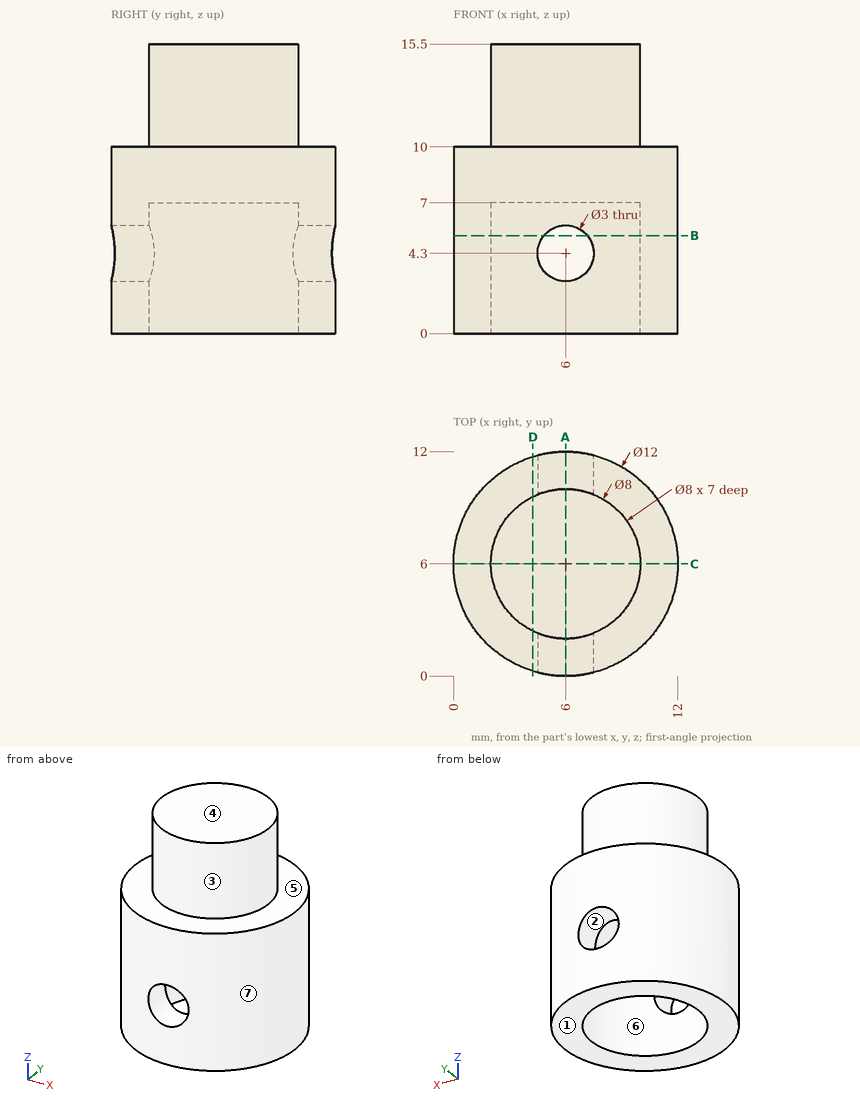
Geometry check sheet. Reference: drawing and pictorial views, mm from the part's lowest x, y, z. A direction names the side the tool comes from. Give positions to 0.01 mm unless a question says otherwise; leave off trailing zeros. Loops run counter-clockwise (first coordinate to the right, second up) from the corner with the lowest first, then second, coordinate; pieces in that order, holes last. Notation, with made-up numbers: M -28,41.5 L -12,41.5 A14 ccw -12,49.5 Z; hole C 41.5,70.5 d8. An arc over 180 degrees is marked long. Use a Markdown table: item, result. Add a question column.
Q1. Sectioned sample at A-A, the plane x = 6. Record the cut outline in (y, z), then the cut area to 3 significant figures.
Q2. Sectioned sample at D-D, the plane x = 4.25. Record the cut outline in (y, z).
Q3. Tool access check on the marked faces 5, 6 and 7. Record the directions out of +Z, -Z, +X, -X, +Y, -Y that give a thin tool (end or side, any length) a straight path to the whole face; none if there is none.
Q4. Go/stop test with flat-tipped pins: pin 1 (4 mm diameter, centred on y = 2.5, z = 9.5, fed in from -X); pin 2 (2.5 mm diameter, centred on x = 4.5, y = 5, fed in from -Z); pin 3 (1 mm diameter, centred on y = 10.5, z = 3, fed in from -X); pin 4 (2.5 mm diameter, centred on x = 6, z = 4.3, fed in from +Y). Record where each tip stops, or that it passes through.
Q5. Scan lines: line 1 along Z through (x, y) = (6, 0.65); line 2 along Z through (x, y) = (7.5, 4); line 3 along Z through (x, y) = (1.75, 9). Record each from-to range of solid material in increasing order. Write a range as [from, to].
Q6. Sectioned sample at C-C, the plane y = 6. Record the cut outline in (x, z), then the cut area to 3 significant figures.
Q7. Mould release check, pull along Z, two halves, no side actions. Record for the marked faces 1, 2, 3 and 4: pulls with the +Z half, pulls with the -Z half, needs draft (parallel to the pull), parting line crosses it, or undercut.
Q8. Sectioned sample at B-B, the plane z = 5.25. Record the cut outline in (x, y).
Verdict:
| question | item | result |
|---|---|---|
| 1 | outline | M 0,0 L 2,0 L 2,2.8 L 0,2.8 Z; M 0,5.8 L 2,5.8 L 2,7 L 10,7 L 10,5.8 L 12,5.8 L 12,10 L 10,10 L 10,15.5 L 2,15.5 L 2,10 L 0,10 Z; M 10,0 L 12,0 L 12,2.8 L 10,2.8 Z |
| 1 | area | 96.0 mm^2 |
| 2 | outline | M 0.26,0 L 2.4,0 L 2.4,7 L 9.6,7 L 9.6,0 L 11.74,0 L 11.74,10 L 9.6,10 L 9.6,15.5 L 2.4,15.5 L 2.4,10 L 0.26,10 Z |
| 3 | face 5 | +Z |
| 3 | face 6 | -Z |
| 3 | face 7 | +Z, -Z |
| 4 | pin 1 | x = 0.19 |
| 4 | pin 2 | z = 7 |
| 4 | pin 3 | x = 1.53 |
| 4 | pin 4 | through |
| 5 | line 1 | [0, 2.8], [5.8, 10] |
| 5 | line 2 | [7, 15.5] |
| 5 | line 3 | [0, 10] |
| 6 | outline | M 0,0 L 2,0 L 2,7 L 10,7 L 10,0 L 12,0 L 12,10 L 10,10 L 10,15.5 L 2,15.5 L 2,10 L 0,10 Z |
| 6 | area | 108 mm^2 |
| 7 | face 1 | pulls with the -Z half |
| 7 | face 2 | undercut |
| 7 | face 3 | needs draft |
| 7 | face 4 | pulls with the +Z half |
| 8 | outline | M 4.84,0.11 L 4.84,2.17 A4 cw 4.84,9.83 L 4.84,11.89 A6 ccw Z; M 7.16,0.11 A6 ccw 7.16,11.89 L 7.16,9.83 A4 cw 7.16,2.17 Z |
